The listing builds one solid part. Answer for the finished solid, in the listing's coordinates (mm). Round coordinates to 2 decimals unless told otherwise and drop trailing zeros. Write each loop counter-clockwise with the first axis right and the second up, starting at its lowest first coordinate (ties: lowest second). Pieces come first, ordered by that corner, then holes. Notation, with made-up numbers: M 47.25,68.25 L 100.25,68.25 A21 cw 100.25,92.25 Z; hole C -8,26 d5. An arc over 180 degrees is marked long. Put each result on its own line as item: value. Start each with the question number.
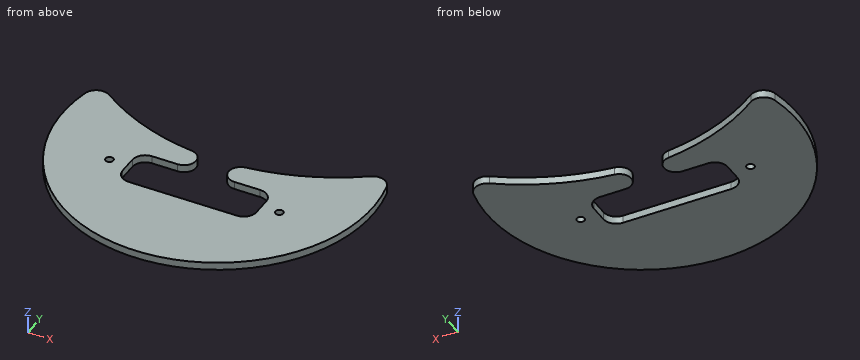
```python
from build123d import *

# Parameters (mm, degrees)
SKETCH1_R           = 1.5
BOSS_EXTRUDE1_DEPTH = 3
FILLET4_R           = 5


with BuildPart() as part:
    # Sketch1 → Boss-Extrude1 (new body)
    with BuildSketch(Plane.XY):
        with BuildLine():
            Line((-25.848592033, 6.75), (26.151407967, 6.75))
            Line((26.151407967, 6.75), (26.151407967, 23.75))
            Line((26.151407967, 23.75), (11.151407967, 23.75))
            ThreePointArc((11.151407967, 23.75), (6.530900978, 28.102570311), (10.600025023, 32.974549649))
            ThreePointArc((10.600025023, 32.974549649), (35.015964593, 39.57666935), (56.532965215, 52.8712086))
            ThreePointArc((56.532965215, 52.8712086), (0.151407967, -27.65), (-56.23014928, 52.8712086))
            ThreePointArc((-56.23014928, 52.8712086), (-34.713148658, 39.57666935), (-10.297209088, 32.974549649))
            ThreePointArc((-10.297209088, 32.974549649), (-6.228085043, 28.102570311), (-10.848592033, 23.75))
            Line((-10.848592033, 23.75), (-25.848592033, 23.75))
            Line((-25.848592033, 23.75), (-25.848592033, 6.75))
        make_face()
        with Locations((-32.848592033, 15.25)):
            Circle(SKETCH1_R, mode=Mode.SUBTRACT)
        with Locations((33.151407967, 15.25)):
            Circle(SKETCH1_R, mode=Mode.SUBTRACT)
    extrude(amount=BOSS_EXTRUDE1_DEPTH)

    # Fillet4
    fillet4_edges = [part.edges().sort_by_distance(p)[0] for p in [
        (-25.848592033, 23.75, 1.5),
        (-25.848592033, 6.75, 1.5),
        (26.151407967, 6.75, 1.5),
        (26.151407967, 23.75, 1.5),
        (56.532965215, 52.8712086, 1.5),
        (-56.23014928, 52.8712086, 1.5),
    ]]
    fillet(fillet4_edges, radius=FILLET4_R)


solid = part.part
```
Item 1: Section D-D (y = -16) is taken. Give the vertices of the cut face in (x, z).
Item 2: Section A-A (y = 15.25) is taken. Give the vertices of the cut face in (x, z), and give its area (3 significant figures).
Item 3: Consider line 1 along Y through (x, z) = (1.5, 2.9); line 2 along X through (y, z) = (26, 0.2); line 3 along X through (y, z) = (18, 1.45). Determine where each line is inside the solid, lowest interval first. Write a range as [from, to].
Item 4: Section B-B (x = 19) is taken. Give the vertices of the cut face in (y, z), and give its area (3 significant figures).
Item 5: Flat-ended cylindrical pins translate along their axes: pin 1 (1.5 mm diameter, centred on y = 15, z = 1.5, fed in from +X); pin 2 (0.9 mm diameter, centred on x = 7.5, z = 1, fed in from +Y); pin 3 (1.5 mm diameter, centred on x = 18, z = 1, fed in from -Y); pin 4 (2.5 mm diameter, centred on x = 33.15, y = 15.25, fed in from -Z). Find the tip coordinate at first contact, or state that the pin passes through.
Item 6: Section C-C (z = 1.6) is taken. Count the separate pieces of the cut face and the enclosed holes in it, and give its area (3 significant figures).
Output values:
1. outline: M -35.38,0 L 35.68,0 L 35.68,3 L -35.38,3 Z
2. outline: M -57.36,0 L -34.35,0 L -34.35,3 L -57.36,3 Z; M -31.35,0 L -25.85,0 L -25.85,3 L -31.35,3 Z; M 26.15,0 L 31.65,0 L 31.65,3 L 26.15,3 Z; M 34.65,0 L 57.66,0 L 57.66,3 L 34.65,3 Z
2. area: 171 mm^2
3. line 1: y = [-27.63, 6.75]
3. line 2: x = [-59.51, -6.88], [7.18, 59.81]
3. line 3: x = [-58.11, -25.85], [26.15, 58.41]
4. outline: M -24.61,0 L 6.75,0 L 6.75,3 L -24.61,3 Z; M 23.75,0 L 34.4,0 L 34.4,3 L 23.75,3 Z
4. area: 126 mm^2
5. pin 1: stops at x = 57.81
5. pin 2: stops at y = 31.72
5. pin 3: stops at y = -25.16
5. pin 4: passes through
6. separate pieces: 1
6. enclosed holes: 2
6. area: 5,460 mm^2
